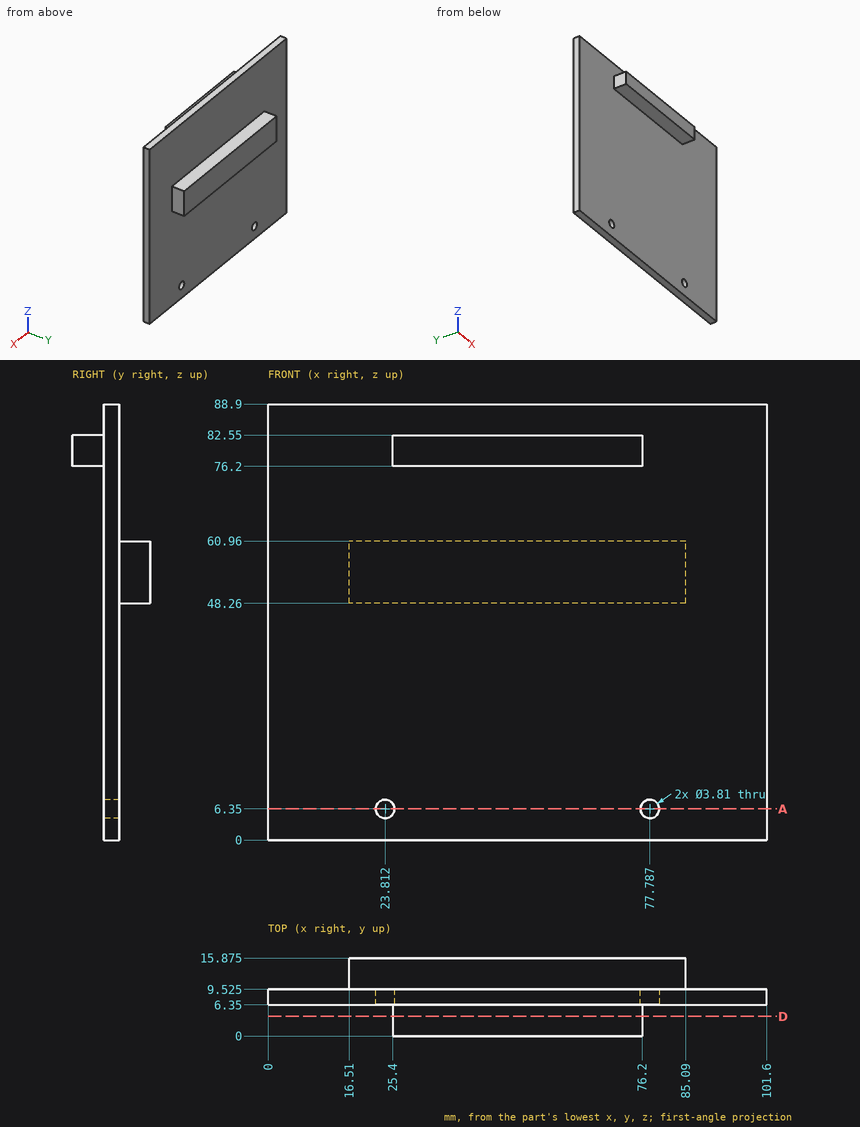
Could you check a few things on this drawing? It's one solid part, dimensions in mm from its lowest x, y, z. Round coordinates to 2 decimals unless told otherwise and drop trailing zeros. Order: outer loops, then holes, each group sorted by start corner. A loop starts at its lowest first (then second) coordinate and runs counter-clockwise, first axis right, second up. Notation, with made-up numbers: M -21,-22 L -7,-22 A20 cw -7,8 Z; hole C -19.5,1.5 d6. An arc over 180 degrees is marked long. Return JSON: item names as keys, results as strings. Group by question number.
1. Please list where these lines run through material, in increasing order: probe 1 along Z at (x, y) = (47, 10); probe 2 along Z at (x, y) = (43, 1); probe 3 along Y at (x, z) = (74, 77) (1 decimal).
2. I'm going to push flat-ended pins straight in: pin 1 Ø6 at (x, z) = (23.81, 6.35) entering from -Y; pin 2 Ø5 at (y, z) = (4, 79) entering from -X; pin 3 Ø4 at (y, z) = (2.5, 68) entering from -X; pin 4 Ø3 at (x, z) = (25.5, 20) entering from +Y (1 decimal). Where does each tip first touch, or does it pass through?
3. If we section it at A-A on z = 6.35: State how many separate pieces and enclosed holes the cut face has.
4. If we section it at D-D on y = 4: List the corners of the cut face in (x, z) for me.
Reply:
{
 "1": {"probe 1": "48.26 to 60.96", "probe 2": "76.2 to 82.55", "probe 3": "0 to 9.5"},
 "2": {"pin 1": "y = 6.35", "pin 2": "x = 0", "pin 3": "through", "pin 4": "y = 9.5"},
 "3": {"separate pieces": "3", "enclosed holes": "0"},
 "4": {"outline": "M 25.4,76.2 L 76.2,76.2 L 76.2,82.55 L 25.4,82.55 Z"}
}
